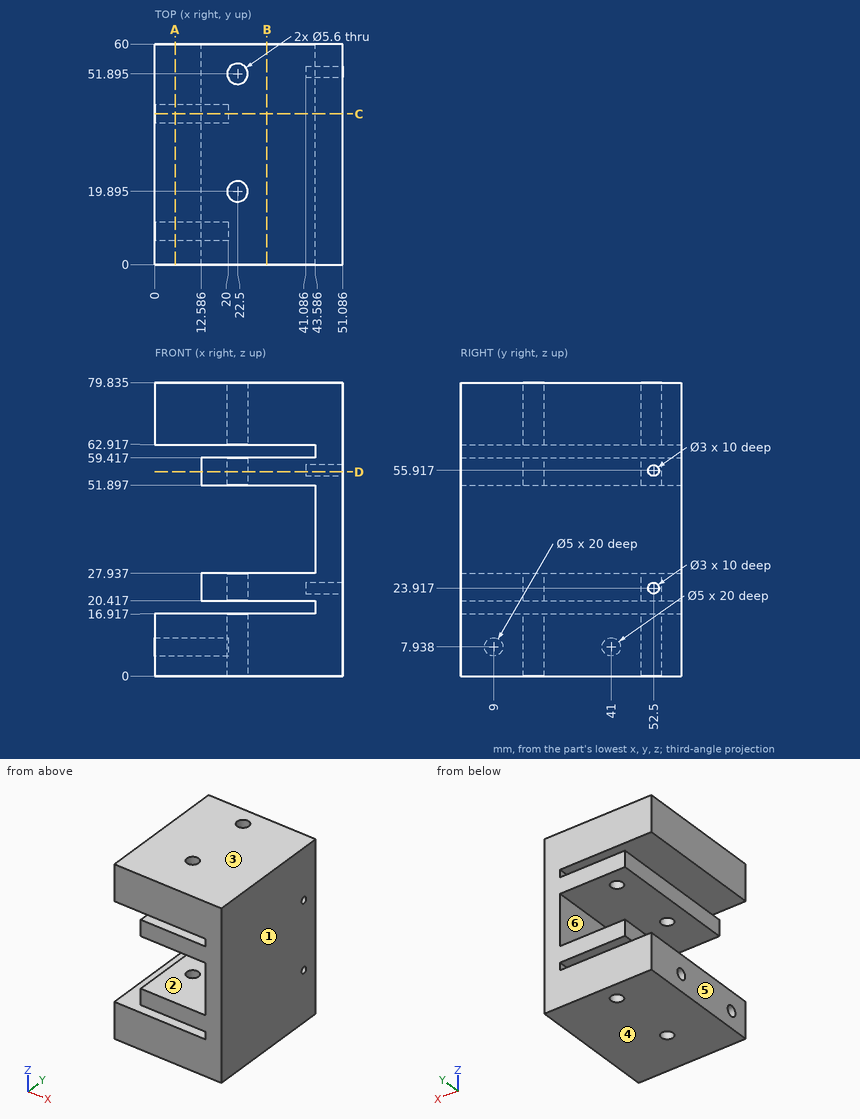
Check sheet for the drawn part. Datum: minimum x, y, z corner. Units: mm. A direction names the side the tool comes from. Round coordinates to 2 decimals unless told otherwise and drop trailing zeros. Loops run counter-clockwise (first coordinate to the right, second up) from the corner with the lowest first, then second, coordinate; pieces in that order, holes last.
Item 1: Cross-section at B-B on x = 30.5. Record the boundary of the cut face in (y, z) (1 decimal).
Item 2: Gauge pin test, flat ends, axial feed: pin 1 (4 mm diameter, centred on y = 52.5, z = 55.92, fed in from -X); pin 2 (5.5 mm diameter, centred on y = 10, z = 7, fed in from -X); pin 3 (2.5 mm diameter, centred on y = 52.5, z = 23.92, fed in from +X); pin 4 (2 mm diameter, centred on y = 52, z = 30.5, fed in from -X). Record the tip position at first contact, or that the pin passes through.
Item 3: Cross-section at A-A on x = 5.5. Record the boundary of the cut face in (y, z) (1 decimal), then the cut area to 3 significant figures.
Item 4: Cross-section at D-D on z = 55.5. Record the boundary of the cut face in (x, y) (1 decimal).
Item 5: Mould release check, pull along Z, two halves, no side actions. Record for the marked faces 1, 2, 3 and 4: pulls with the +Z half, pulls with the -Z half, needs draft (parallel to the pull), parting line crosses it, or undercut.
Item 6: Access from +Z, -Z, +X, -X, +Y, -Y to the whole of each face (thin tool, end or side, straight path). Record for the marked faces 5 and 6.
Item 7: Thickness scan on line 1 (Y direction, x = 22.5, z = 5) (1 decimal); line 2 (Z direction, x = 35.5, y = 55) (1 decimal); line 3 (Z direction, x = 11.5, y = 46.5) (1 decimal). Record the ranges inside material, lowest first.
Item 8: Cross-section at C-C on y = 41. Record the boundary of the cut face in (x, z) (1 decimal).
Answer sheet:
1. outline: (0, 0) - (60, 0) - (60, 16.9) - (0, 16.9) - close; (0, 20.4) - (60, 20.4) - (60, 27.9) - (0, 27.9) - close; (0, 51.9) - (60, 51.9) - (60, 59.4) - (0, 59.4) - close; (0, 62.9) - (60, 62.9) - (60, 79.8) - (0, 79.8) - close
2. pin 1: stops at x = 12.59
2. pin 2: stops at x = 0
2. pin 3: stops at x = 41.09
2. pin 4: stops at x = 43.59
3. outline: (0, 0) - (60, 0) - (60, 16.9) - (0, 16.9) - close; (0, 62.9) - (60, 62.9) - (60, 79.8) - (0, 79.8) - close; hole circle Ø5 at (9, 7.9); hole circle Ø5 at (41, 7.9)
3. area: 1,990 mm2
4. outline: (12.6, 0) - (51.1, 0) - (51.1, 51.1) - (41.1, 51.1) - (41.1, 53.9) - (51.1, 53.9) - (51.1, 60) - (12.6, 60) - close; hole circle Ø5.6 at (22.5, 19.9); hole circle Ø5.6 at (22.5, 51.9)
5. face 1: needs draft
5. face 2: undercut
5. face 3: pulls with the +Z half
5. face 4: pulls with the -Z half
6. face 5: +Z, -Z, -X, +Y, -Y
6. face 6: -X, +Y, -Y
7. line 1: y = 0 to 17.1, 22.7 to 49.1, 54.7 to 60
7. line 2: z = 0 to 16.9, 20.4 to 27.9, 51.9 to 59.4, 62.9 to 79.8
7. line 3: z = 0 to 16.9, 62.9 to 79.8
8. outline: (0, 0) - (51.1, 0) - (51.1, 79.8) - (0, 79.8) - (0, 62.9) - (43.6, 62.9) - (43.6, 59.4) - (12.6, 59.4) - (12.6, 51.9) - (43.6, 51.9) - (43.6, 27.9) - (12.6, 27.9) - (12.6, 20.4) - (43.6, 20.4) - (43.6, 16.9) - (0, 16.9) - (0, 10.4) - (20, 10.4) - (20, 5.4) - (0, 5.4) - close
